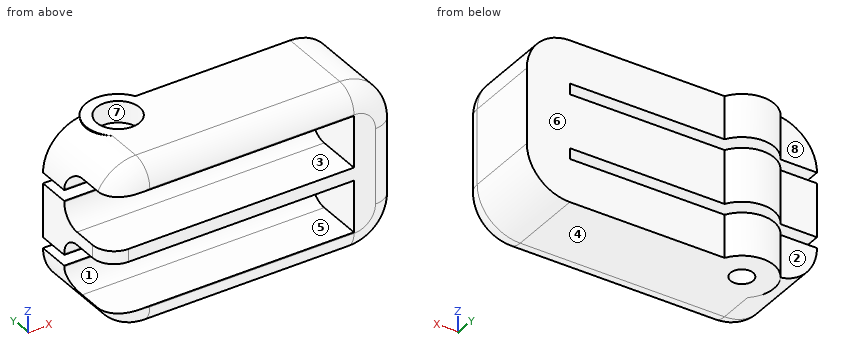
```python
from build123d import *

# Parameters (mm, degrees)
CYLINDER002_R          = 2
CYLINDER002_DEPTH      = 2
CYLINDER_R             = 1.05
CYLINDER_DEPTH         = 20
CYLINDER_ROLL_ANGLE    = 90
RECTANGLE004_W         = 26
RECTANGLE004_H         = 4.8
EXTRUDE005_DEPTH       = 8
RECTANGLE002_W         = 26
RECTANGLE002_H         = 1
EXTRUDE004_DEPTH       = 20
RECTANGLE005_W         = 26
RECTANGLE005_H         = 4.8
EXTRUDE008_DEPTH       = 8
RECTANGLE001_W         = 26
RECTANGLE001_H         = 1
EXTRUDE002_DEPTH       = 20
RECTANGLE_W            = 27
RECTANGLE_H            = 15
EXTRUDE_DEPTH          = 9
FILLET_R               = 4
FILLET001_R            = 1.8
RECTANGLE008_W         = 26
RECTANGLE008_H         = 4.8
EXTRUDE011_DEPTH       = 8
RECTANGLE007_W         = 26
RECTANGLE007_H         = 1
EXTRUDE010_DEPTH       = 20
RECTANGLE009_W         = 26
RECTANGLE009_H         = 4.8
EXTRUDE012_DEPTH       = 8
RECTANGLE006_W         = 26
RECTANGLE006_H         = 1
EXTRUDE009_DEPTH       = 20
CYLINDER001_R          = 3
CYLINDER001_DEPTH      = 15
CYLINDER001_ROLL_ANGLE = 90
CUT002_ROLL_ANGLE      = 90
FILLET002_R            = 2


with BuildPart() as cylinder002:
    # Cylinder002 → Cylinder002 (new body)
    with BuildSketch(Plane(origin=(-14, -1.5, 18), x_dir=(1, 0, 0), z_dir=(0, 0, 1))):
        Circle(CYLINDER002_R)
    extrude(amount=CYLINDER002_DEPTH)


with BuildPart() as cylinder:
    # Cylinder → Cylinder (new body)
    with BuildSketch(Plane.XY):
        Circle(CYLINDER_R)
    extrude(amount=CYLINDER_DEPTH)


with BuildPart() as cylinder_1:
    # Cylinder roll: moved
    add(cylinder.part.rotate(Axis((0, 0, 0), (1, 0, 0)), CYLINDER_ROLL_ANGLE))


with BuildPart() as cylinder_2:
    # Cylinder placement: moved
    add(cylinder_1.part.moved(Location((-14, 21, 1.5))))


with BuildPart() as extrude005:
    # Rectangle004 → Extrude005 (new body)
    with BuildSketch(Plane(origin=(-23, 13.1, 0), x_dir=(1, 0, 0), z_dir=(0, 0, 1))):
        with Locations((13, 2.4)):
            Rectangle(RECTANGLE004_W, RECTANGLE004_H)
    extrude(amount=-EXTRUDE005_DEPTH)


with BuildPart() as extrude005_1:
    # Extrude005 placement: moved
    add(extrude005.part.moved(Location((0, 0, 11))))


with BuildPart() as extrude004:
    # Rectangle002 → Extrude004 (new body)
    with BuildSketch(Plane(origin=(-23, 10, 0), x_dir=(1, 0, 0), z_dir=(0, 0, 1))):
        with Locations((13, -0.5)):
            Rectangle(RECTANGLE002_W, RECTANGLE002_H)
    extrude(amount=EXTRUDE004_DEPTH)


with BuildPart() as extrude004_1:
    # Extrude004 placement: moved
    add(extrude004.part.moved(Location((0, 0, -4))))


with BuildPart() as extrude008:
    # Rectangle005 → Extrude008 (new body)
    with BuildSketch(Plane(origin=(-23, 11.9, 0), x_dir=(1, 0, 0), z_dir=(0, 0, 1))):
        with Locations((13, -2.4)):
            Rectangle(RECTANGLE005_W, RECTANGLE005_H)
    extrude(amount=EXTRUDE008_DEPTH)


with BuildPart() as extrude008_1:
    # Extrude008 placement: moved
    add(extrude008.part.moved(Location((0, 0, 3))))


with BuildPart() as fusion:
    # Rectangle001 → Extrude002 (new body)
    with BuildSketch(Plane(origin=(-23, 16, 0), x_dir=(1, 0, 0), z_dir=(0, 0, 1))):
        with Locations((13, 0.5)):
            Rectangle(RECTANGLE001_W, RECTANGLE001_H)
    extrude(amount=-EXTRUDE002_DEPTH)


with BuildPart() as fusion_1:
    # Extrude002 placement: moved
    add(fusion.part.moved(Location((0, -1, 10))))

    # Fusion: union Extrude005, Extrude004, Extrude008
    add(extrude005_1.part)
    add(extrude004_1.part)
    add(extrude008_1.part)


with BuildPart() as fillet001:
    # Rectangle → Extrude (new body)
    with BuildSketch(Plane(origin=(-20, 20, 0), x_dir=(1, 0, 0), z_dir=(0, 0, 1))):
        with Locations((13.5, -7.5)):
            Rectangle(RECTANGLE_W, RECTANGLE_H)
    extrude(amount=EXTRUDE_DEPTH)

    # Fillet
    fillet_edges = [fillet001.edges().sort_by_distance(p)[0] for p in [
        (-20, 20, 4.5),
        (7, 20, 4.5),
        (7, 5, 4.5),
        (-20, 5, 4.5),
    ]]
    fillet(fillet_edges, radius=FILLET_R)

    # Cut: cut Fusion
    add(fusion_1.part, mode=Mode.SUBTRACT)

    # Fillet001
    fillet001_edges = [fillet001.edges().sort_by_distance(p)[0] for p in [
        (-8.259972, 17.9, 3),
        (-8.259972, 7.1, 3),
        (-8.5, 11.9, 3),
        (-8.5, 13.1, 3),
    ]]
    fillet(fillet001_edges, radius=FILLET001_R)


with BuildPart() as extrude011:
    # Rectangle008 → Extrude011 (new body)
    with BuildSketch(Plane(origin=(-23, 13.1, 0), x_dir=(1, 0, 0), z_dir=(0, 0, 1))):
        with Locations((13, 2.4)):
            Rectangle(RECTANGLE008_W, RECTANGLE008_H)
    extrude(amount=-EXTRUDE011_DEPTH)


with BuildPart() as extrude011_1:
    # Extrude011 placement: moved
    add(extrude011.part.moved(Location((0, 0, 11))))


with BuildPart() as extrude010:
    # Rectangle007 → Extrude010 (new body)
    with BuildSketch(Plane(origin=(-23, 10, 0), x_dir=(1, 0, 0), z_dir=(0, 0, 1))):
        with Locations((13, -0.5)):
            Rectangle(RECTANGLE007_W, RECTANGLE007_H)
    extrude(amount=EXTRUDE010_DEPTH)


with BuildPart() as extrude010_1:
    # Extrude010 placement: moved
    add(extrude010.part.moved(Location((0, 0, -4))))


with BuildPart() as extrude012:
    # Rectangle009 → Extrude012 (new body)
    with BuildSketch(Plane(origin=(-23, 11.9, 0), x_dir=(1, 0, 0), z_dir=(0, 0, 1))):
        with Locations((13, -2.4)):
            Rectangle(RECTANGLE009_W, RECTANGLE009_H)
    extrude(amount=EXTRUDE012_DEPTH)


with BuildPart() as extrude012_1:
    # Extrude012 placement: moved
    add(extrude012.part.moved(Location((0, 0, 3))))


with BuildPart() as fusion001:
    # Rectangle006 → Extrude009 (new body)
    with BuildSketch(Plane(origin=(-23, 16, 0), x_dir=(1, 0, 0), z_dir=(0, 0, 1))):
        with Locations((13, 0.5)):
            Rectangle(RECTANGLE006_W, RECTANGLE006_H)
    extrude(amount=-EXTRUDE009_DEPTH)


with BuildPart() as fusion001_1:
    # Extrude009 placement: moved
    add(fusion001.part.moved(Location((0, -1, 10))))

    # Fusion001: union Extrude011, Extrude010, Extrude012
    add(extrude011_1.part)
    add(extrude010_1.part)
    add(extrude012_1.part)


with BuildPart() as fillet002:
    # Cylinder001 → Cylinder001 (new body)
    with BuildSketch(Plane.XY):
        Circle(CYLINDER001_R)
    extrude(amount=CYLINDER001_DEPTH)


with BuildPart() as fillet002_1:
    # Cylinder001 roll: moved
    add(fillet002.part.rotate(Axis((0, 0, 0), (1, 0, 0)), CYLINDER001_ROLL_ANGLE))


with BuildPart() as fillet002_2:
    # Cylinder001 placement: moved
    add(fillet002_1.part.moved(Location((-14, 20, 1.5))))

    # Cut001: cut Fusion001
    add(fusion001_1.part, mode=Mode.SUBTRACT)

    # Fusion002: union Fillet001
    add(fillet001.part)

    # Cut002: cut Cylinder
    add(cylinder_2.part, mode=Mode.SUBTRACT)


with BuildPart() as fillet002_3:
    # Cut002 roll: moved
    add(fillet002_2.part.rotate(Axis((0, 0, 0), (1, 0, 0)), CUT002_ROLL_ANGLE))


with BuildPart() as fillet002_4:
    # Cut002 placement: moved
    add(fillet002_3.part)

    # Cut003: cut Cylinder002
    add(cylinder002.part, mode=Mode.SUBTRACT)

    # Fillet002
    fillet002_edges = [fillet002_4.edges().sort_by_distance(p)[0] for p in [
        (-6.5, -9, 20),
        (5.828427, -9, 18.828427),
        (7, -9, 12.5),
        (5.828427, -9, 6.171573),
        (-6.5, -9, 5),
        (-18.04939, -9, 5.564887),
        (-20, -9, 12.5),
        (-18.04939, -9, 19.435113),
    ]]
    fillet(fillet002_edges, radius=FILLET002_R)


solid = fillet002_4.part
```
Model file for the job. Use its own axes, mm. Face numbers are marked on the shaded views. A direction names the side the tool comes from. Coordinates: 2 decimals unless noted, no trailing zeros. Order: outer loops, then holes, each group sorted by start corner. A loop starts at its lowest first (then second) coordinate and runs counter-clockwise, first axis right, second up. Notation, with made-up numbers: (-5.75, 81.5) - (43.25, 81.5) arc R5 cw to (43.25, 89.5) - close; hole circle Ø6 at (34.5, 86). An arc over 180 degrees is marked (long way). Return JSON: item names as keys, results as strings. Group by question number.
1) Tool access for the marked faces 5, 6, 7 and 8: list every direction of +Z, -Z, +X, -X, +Y, -Y with a clear straight run to the whole face (end or side of a thin tool).
2) Flat gauge pins, fed straight in: P1, Ø2.5, axis at x = -14, y = -1.5, coming from the +Z side; P2, Ø1, axis at x = -3.5, z = 16, coming from the -Y side (3 decimals); P3, Ø1, axis at x = -17.5, z = 17, coming from the +Y side. Where does each tip first touch, or does it go through?
3) Saw through at A-A, the plane x = -3.25. Write the cut outline in (y, z), plus the area to 3 significant figures.
4) Saw through at C-C, the plane z = 13.75. Write the cut outline in (x, y), plus the area to 3 significant figures.
5) Probe line 1 (Z direction, x = -4.25, y = -6.5); line 2 (Z direction, x = -2, y = -1.5); line 3 (Y direction, x = -1, z = 12). List the from-to ranges inside material, lowest first. Write a range as from..to.
6) Mould opens along Z. For the marked faces 1, 2, 3 and 4 say: released by +Z, released by -Z, zero draft, split by the parting line, or undercut.
7) Saw through at B-B, the plane y = -1.5. Count the separate pieces of the cut face and the enclosed holes in it, plus the area to 3 significant figures.
Values found:
{
 "1": {"face 5": "-X, -Y", "face 6": "+Z, -Z, +X, +Y", "face 7": "+Z", "face 8": "+Z, -Z, -X, +Y"},
 "2": {"P1": "stops at z = 18", "P2": "stops at y = -3.045", "P3": "stops at y = 0"},
 "3": {"outline": "(-9, 7) arc R2 ccw to (-7, 5) - (0, 5) - (0, 9) - (-3, 9) - (-3, 8.9) arc R1.8 cw to (-4.8, 7.1) - (-9, 7.1) - close; (-9, 11.9) - (-4.8, 11.9) arc R1.8 cw to (-3, 10.1) - (-3, 10) - (0, 10) - (0, 15) - (-3, 15) - (-3, 14.9) arc R1.8 cw to (-4.8, 13.1) - (-9, 13.1) - close; (-9, 17.9) - (-4.8, 17.9) arc R1.8 cw to (-3, 16.1) - (-3, 16) - (0, 16) - (0, 20) - (-7, 20) arc R2 ccw to (-9, 18) - close", "area": "72.5 mm²"},
 "4": {"outline": "(-20, -3.42) - (3, -3.42) - (3, -9) - (5, -9) arc R2 ccw to (7, -7) - (7, 0) - (-11.4, 0) arc R3 ccw to (-16.6, 0) - (-20, 0) - close; hole circle Ø2.1 at (-14, -1.5)", "area": "116 mm²"},
 "5": {"line 1": "z = 5..7.1, 11.9..13.1, 17.9..20", "line 2": "z = 5..9, 10..15, 16..20", "line 3": "y = -9..0"},
 "6": {"face 1": "undercut", "face 2": "zero draft", "face 3": "undercut", "face 4": "released by -Z"},
 "7": {"separate pieces": "4", "enclosed holes": "0", "area": "314 mm²"}
}
